Here's how the part is built. I have some questions about the finished solid (model axes, mm). Face numbers are marked on the shaded views. A direction names the side the tool comes from. Round coordinates to 2 decimals unless told otherwise and drop trailing zeros. Write each loop counter-clockwise with the first axis right and the second up, starting at its lowest first coordinate (ties: lowest second). Pieces come first, ordered by that corner, then holes. Notation, with made-up numbers: (-5.5, 56) -> (31.5, 56) arc R20 ccw to (31.5, 91) -> close; hole circle Ø7 at (83.5, -11). An arc over 180 degrees is marked (long way). Put each result on its own line as item: value. Start each with the question number.
1) Which directions (+Z, -Z, +X, -X, +Y, -Y) give clear straight access to the entire face, cutting with the end or side of a thin tool? Please do the marked faces 4, 5, 6 and 7.
2) Will this pin go through, and if not, where does the flat tip stop? P1, Ø1, axis at y = -4, z = 3, coming from the +X side.
3) We'd pull the mould along X, two halves only. Please class the marked faces 1, 2 and 3: released by +X, released by -X, zero draft, split by the parting line, or undercut.
4) If I drill on line 1 along Y through (x, z) = (5, 2.45); line 2 along Y through (x, z) = (4.75, 1.55); line 3 along X through (y, z) = (-5.75, 0.75), over which ranges is the centre line in solid material (lowest first)? Write a range as [from, to].
5) I want a section at A-A, the plane x = -6.5. List the corners of the cut face in (y, z) for me.
6) I want a section at B-B, the plane y = -1.5. List the corners of the cut face in (x, z) for me, then the cut area to 3 significant figures.
7) I want a section at C-C, the plane x = -1. List the corners of the cut face in (y, z) for me.
Autodesk Inventor part; units mm, degrees
ref_plane "Work Plane2" through (0, 0, 2.5) normal (0, 0, 1) x (1, 0, 0)
ref_plane "Work Plane8" through (0, 0, 0) normal (0.9510565, 0.309017, 0) x (0, 0, 1)
ref_plane "Work Plane9" through (0, 0, 0) normal (1, 0, 0) x (0, 1, 0)
sketch "Sketch1" plane through (0, 0, 0) normal (0, 0, 1) x (1, 0, 0)
  circle A0 centre (0, 0) radius 8.9931
  dimension "d0" = 17.9863
extrude "Extrusion1" add sketch "Sketch1" along normal blind 5
ref_plane "Work Plane2" through (0, 0, 2.5) normal (0, 0, 1) x (1, 0, 0)
sketch "Sketch2" plane through (0, 0, 0) normal (0, 0, -1) x (-1, 0, 0)
  circle A0 centre (0, 0) radius 8.9931
  circle A1 centre (0, 0) radius 7.5
  dimension "d3" = 15
surface extrude "Средний диаметр" sketch "Sketch2" against normal through all shown no curves A1
ref_plane "Work Plane8" through (0, 0, 0) normal (0.9510565, 0.309017, 0) x (0, 0, 1)
ref_plane "Work Plane9" through (0, 0, 0) normal (1, 0, 0) x (0, 1, 0)
spur gear teeth "Цилиндрическое зубчатое зацепление" teeth 10 pitch diameter 15 tip diameter 17.9863 root diameter 11.25 face width 5 start plane through (0, 0, 0) normal (0, 0, -1) x (-1, 0, 0)
equation "\"d0\" = da_da"
equation "\"d1\" = da_b"
equation "\"d3\" = da_d"
equation "\"d16\" = da_aw"
equation "\"d43\" = da_aw"
equation "\"d46\" = da_aw"
properties part number "Цилиндрическое зубчатое зацепление1" material "Steel"
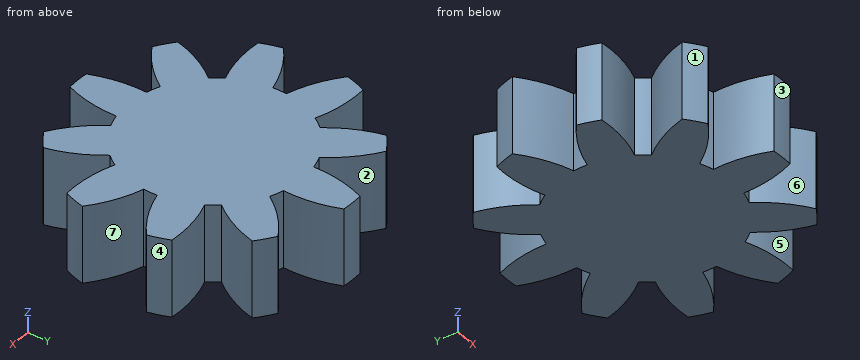
Findings:
1. face 4: +Z, -Z, +X, +Y
1. face 5: +Z, -Z
1. face 6: +Z, -Z, -Y
1. face 7: +Z, -Z, +X
2. P1: stops at x = 4.87
3. face 1: released by -X
3. face 2: undercut
3. face 3: split by the parting line
4. line 1: y = [-7.48, -4.72], [-3.01, 3.01], [4.72, 7.48]
4. line 2: y = [-7.64, -4.31], [-3.01, 3.01], [4.31, 7.64]
4. line 3: x = [-5.49, -2.55], [-1.32, 1.32], [2.55, 5.49]
5. outline: (-3.38, 0) -> (-0.74, 0) -> (-0.74, 5) -> (-3.38, 5) -> close; (0.74, 0) -> (3.38, 0) -> (3.38, 5) -> (0.74, 5) -> close
6. outline: (-7.95, 0) -> (7.95, 0) -> (7.95, 5) -> (-7.95, 5) -> close
6. area: 79.5 mm2
7. outline: (-8.12, 0) -> (8.12, 0) -> (8.12, 5) -> (-8.12, 5) -> close
